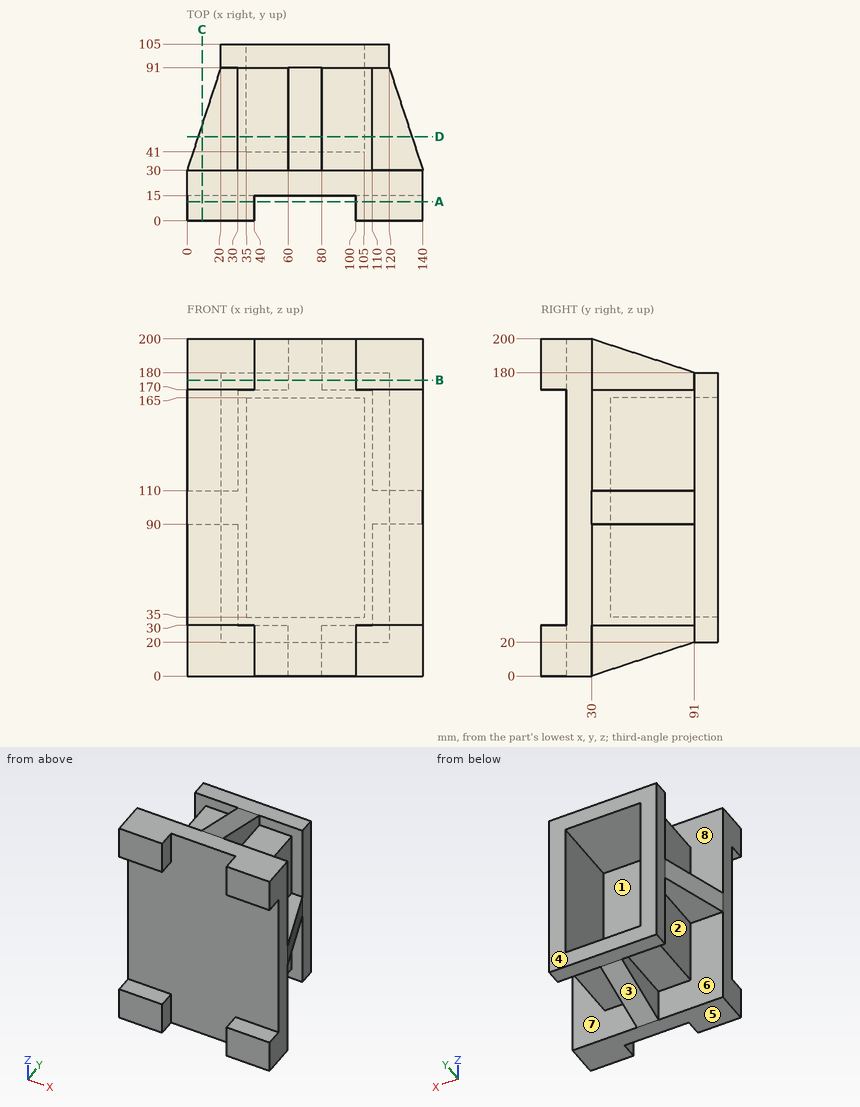
Part print with two shaded views. Sizes in mm from the minimum x, y, z corner. A direction names the side the tool comes from. Coordinates: 2 decimals unless noted, no trailing zeros. Write each loop counter-clockwise with the first axis right and the second up, starting at its lowest first coordinate (ties: lowest second). Pieces come first, ordered by that corner, then holes. Notation, with made-up numbers: M 40.5,-28.75 L 67.5,-28.75 A25 cw 67.5,-14.75 Z; hole C -23,72 d2. An arc over 180 degrees is marked long. Return JSON: item names as keys, results as strings.
Item 1: Two-plate mould, pull along Z, no slides. Class the marked faces 1, 2 and 3: +Z half, -Z half, draft (parallel to the pull), parting line (faces both ways), or undercut.
Findings below:
{"face 1": "undercut", "face 2": "draft", "face 3": "-Z half"}
Item 2: Drop flat-ended pins along their axis: pin 1 Ø10 at (x, z) = (96.5, 137) entering from -Y; pin 2 Ø9 at (y, z) = (54.5, 179) entering from +X; pin 3 Ø9 at (x, y) = (45.5, 63.5) entering from -Z. Give the stop position or say it passes through.
Findings below:
{"pin 1": "stops at y = 15", "pin 2": "stops at x = 80", "pin 3": "stops at z = 30"}
Item 3: Probe line 1 (Z direction, x = 71, y = 98); line 2 (X direction, y = 48, z = 154); line 3 (Z direction, x = 56, y = 86). List the from-to ranges inside material, lowest first. Write a range as from..to.
Findings below:
{"line 1": "z = 20..35, 165..180", "line 2": "x = 30..35, 105..110", "line 3": "z = 30..35, 165..170"}
Item 4: Slice it at D-D, the plane y = 50. Write the cut outline in (x, z), and give its area (3 significant figures).
Findings below:
{"outline": "M 6.56,90 L 30,90 L 30,30 L 60,30 L 60,6.56 L 80,6.56 L 80,30 L 110,30 L 110,90 L 133.44,90 L 133.44,110 L 110,110 L 110,170 L 80,170 L 80,193.44 L 60,193.44 L 60,170 L 30,170 L 30,110 L 6.56,110 Z; hole M 35,35 L 105,35 L 105,165 L 35,165 Z", "area": "3,980 mm2"}
Item 5: Slice it at A-A, the plane y = 11.5. Write the cut outline in (x, z), and give its area (3 significant figures).
Findings below:
{"outline": "M 0,0 L 40,0 L 40,30 L 0,30 Z; M 0,170 L 40,170 L 40,200 L 0,200 Z; M 100,0 L 140,0 L 140,30 L 100,30 Z; M 100,170 L 140,170 L 140,200 L 100,200 Z", "area": "4,800 mm2"}
Item 6: Slice it at C-C, the plane x = 9. Write the cut outline in (y, z), and give its area (3 significant figures).
Findings below:
{"outline": "M 0,0 L 30,0 L 30,90 L 57.45,90 L 57.45,110 L 30,110 L 30,200 L 0,200 L 0,170 L 15,170 L 15,30 L 0,30 Z", "area": "4,450 mm2"}
Item 7: Which spindle directions (+Z, -Z, +X, -X, +Y, -Y) get a long thin tool onto all of the face, cutting with end or side? Do the marked faces 4, 5, 6, 7 and 8. Say none if no direction does.
Findings below:
{"face 4": "+Z, -Z, +X, -X, +Y", "face 5": "-Z, +X, -X, +Y, -Y", "face 6": "-Z, -X", "face 7": "-Z, +X", "face 8": "+Z, -X"}
Item 8: Slice it at B-B, the plane z = 175.5. Write the cut outline in (x, y).
Findings below:
{"outline": "M 0,0 L 40,0 L 40,15 L 100,15 L 100,0 L 140,0 L 140,30 L 80,30 L 80,91 L 120,91 L 120,105 L 20,105 L 20,91 L 60,91 L 60,30 L 0,30 Z"}
